```python
from build123d import *

# Parameters (mm, degrees)
CHAMFER1_SIZE               = 0.381
F_32_0_116_DIAMETER_HOLE1_D = 2.9464
CHAMFER2_SIZE               = 2.032


with BuildPart() as part:
    # Sketch1 → Revolve1 (revolve)
    with BuildSketch(Plane(origin=(0, 0, 0), x_dir=(0, 0, -1), z_dir=(1, 0, 0)), mode=Mode.PRIVATE) as revolve1_sk:
        Polygon((0, 14.1605), (4.7752, 14.1605), (4.7752, 5.5626), (11.684, 5.5626), (11.684, 0), (10.760342906, 0), (8.3566, 4.0005), (-1.1684, 4.0005), (-1.1684, 5.5372), (0, 5.5372), align=None)
    revolve(revolve1_sk.sketch.rotate(Axis((0, 0, -14.800465311), (0, 0, -1)), 90), axis=Axis((0, 0, -14.800465311), (0, 0, -1)))

    # Chamfer1
    chamfer1_edges = [part.edges().sort_by_distance(p)[0] for p in [
        (-14.1605, 0, -4.7752),
        (-14.1605, 0, 0),
    ]]
    chamfer(chamfer1_edges, length=CHAMFER1_SIZE)

    # #32 (0.116) Diameter Hole1 (through all)
    with Locations(Plane(origin=(0, 0, -4.7752), x_dir=(-1, 0, 0), z_dir=(0, 0, -1))):
        with Locations((0, 9.525), (0, -9.525)):
            Hole(F_32_0_116_DIAMETER_HOLE1_D / 2)

    # Chamfer2
    chamfer2_edges = [part.edges().sort_by_distance(p)[0] for p in [
        (-5.5626, 0, -11.684),
    ]]
    chamfer(chamfer2_edges, length=CHAMFER2_SIZE)


solid = part.part
```
The model under review builds one solid part; all positions refer to its coordinate system, in mm. A direction names the side the tool comes from. Round coordinates to 2 decimals unless told otherwise and drop trailing zeros. Order: outer loops, then holes, each group sorted by start corner. A loop starts at its lowest first (then second) coordinate and runs counter-clockwise, first axis right, second up.
(1) For P1, Ø4, axis at x = 9.5, y = -3.5, coming from the -Z side; P2, Ø1.5, axis at x = -9.5, z = -7, coming from the -Y side; P3, Ø5, axis at x = 0, y = 0, coming from the +Z side; P4, Ø5, axis at x = -6.5, z = -10, coming from the +Y side, all flat-tipped, find the tip position at first contact; note any pin that passes through.
Working result:
P1: stops at z = -4.78
P2: passes through
P3: stops at z = -9.26
P4: stops at y = 3.84
(2) Wall thickness on L1, parallel to Y at x = 0, z = -0.95; L2, parallel to Z at x = -4, y = -10.5; L3, parallel to X at y = 1.5, z = -4.5: over which ranges is each line inside the solid? List them lowest first.
Working result:
L1: y = -14.16 to -11, -8.05 to -4, 4 to 8.05, 11 to 14.16
L2: z = -4.78 to 0
L3: x = -13.97 to -3.71, 3.71 to 13.97
(3) Tool access review of faces 4 (the face through (0, 0, -11.684)), 5 (the face through (-0.9, 3.9, -3.5)), 6 (the face through (5.306, -1.671, -7.248)): name each direction out of +Z, -Z, +X, -X, +Y, -Y from which nothing blocks a thin tool from reaching the whole face with its end or side.
Working result:
face 4: -Z, +X, -X, +Y, -Y
face 5: +Z
face 6: -Z
(4) Mouldability with a two-part tool opening along Y and no side actions: class faces 1 (the face through (0, 6, -4.775)), 2 (the face through (-1.84, -14.04, -2.42)), 3 (the face through (-0.192, -8.064, -2.354)) as released by +Y, released by -Y, zero draft, split by the parting line, or undercut.
Working result:
face 1: zero draft
face 2: split by the parting line
face 3: undercut
(5) Take a section at A-A, the plane z = -7.5. State the section outline as (x, y) points, plus the area to 3 significant figures.
Working result:
outline: circle Ø11.13 at (0, 0); hole circle Ø8 at (0, 0)
area: 46.9 mm2
(6) Take a section at B-B, the plane z = -1.25. State the section outline as (x, y) points (1 decimal), plus the area to 3 significant figures.
Working result:
outline: circle Ø28.3 at (0, 0); hole circle Ø8 at (0, 0); hole circle Ø2.9 at (0, -9.5); hole circle Ø2.9 at (0, 9.5)
area: 566 mm2
